Input: part model. Units: mm. Frame: model coordinates. A direction names the side the tool comes from. Coordinates: 2 decimals unless noted, no trailing zeros. Loops run counter-clockwise (first coordinate to the right, second up) from the corner with the lowest first, then second, coordinate; pieces in that order, holes last. Notation, with made-up numbers: (1, 16.5) - (26, 16.5) arc R19 ccw to (26, 26.5) - close; hole circle Ø4 at (83.25, -29.5). An arc over 180 degrees is marked (long way). Use one line per item in the form item = value.
from build123d import *

# Parameters (mm, degrees)
F0_W     = 660.4
F0_H     = 254
F1_DEPTH = 152.4
F2_W     = 654.05
F2_H     = 247.65
F3_DEPTH = 152.401
F4_W     = 685.8
F4_H     = 279.4
F4_W_2   = 660.4
F4_H_2   = 254
F5_DEPTH = 3.175
F6_R     = 9.525
F7_DEPTH = 3.175


with BuildPart() as f1:
    # F0 (on Top) → F1 (new body)
    with BuildSketch(Plane.XY):
        Rectangle(F0_W, F0_H)
    extrude(amount=F1_DEPTH)

    # F2 (on face) → F3 (cut, through all)
    with BuildSketch(Plane.XY.offset(152.4)):
        Rectangle(F2_W, F2_H)
    extrude(amount=-F3_DEPTH, mode=Mode.SUBTRACT)

    # F4 (on face) → F5 (join)
    with BuildSketch(Plane.XY.offset(152.4)):
        Rectangle(F4_W, F4_H)
        Rectangle(F4_W_2, F4_H_2, mode=Mode.SUBTRACT)
    extrude(amount=-F5_DEPTH)

    # F6 (on face) → F7 (cut, through all)
    with BuildSketch(Plane.XZ.offset(127)):
        with Locations((0, 25.4)):
            Circle(F6_R)
    extrude(amount=-F7_DEPTH, mode=Mode.SUBTRACT)


solid = f1.part
Q1. Set-up query: faces 1 (the flat face through (-5, 127, 74)), 2 (the flat face through (330.2, -2, 74)), 3 (the cylindrical face through (-2.06, -125.43, 16.1)), 4 (the flat face through (-327.025, -2, 77)). Return all of +Z, -Z, +X, -X, +Y, -Y with unobstructed straight access to the full face (end or side cutting, diameter ignored); none if empty.
Check values:
face_1 = -Z, +X, -X, +Y
face_2 = -Z, +X, +Y, -Y
face_3 = -Y
face_4 = +Z, -Z
Q2. Cut plane C-C, the plane x = 0. Return loops of the section in (y, z) (3 decimals).
Check values:
outline = (-139.7, 149.225) - (-127, 149.225) - (-127, 34.925) - (-123.825, 34.925) - (-123.825, 152.4) - (-139.7, 152.4) - close; (-127, 0) - (-123.825, 0) - (-123.825, 15.875) - (-127, 15.875) - close; (123.825, 0) - (127, 0) - (127, 149.225) - (139.7, 149.225) - (139.7, 152.4) - (123.825, 152.4) - close
Q3. Cut plane A-A, the plane y = 95. Return loops of the section in (x, z) (3 decimals).
Check values:
outline = (-342.9, 149.225) - (-330.2, 149.225) - (-330.2, 0) - (-327.025, 0) - (-327.025, 152.4) - (-342.9, 152.4) - close; (327.025, 0) - (330.2, 0) - (330.2, 149.225) - (342.9, 149.225) - (342.9, 152.4) - (327.025, 152.4) - close
Q4. Ray query, line 1 along Y through (x, z) = (76, 49.5) (3 decimals); line 2 along X through (y, z) = (-20, 90.5) (3 decimals); line 3 along Z through (x, y) = (0, -124.75) (3 decimals). Return the intervals inside material, ascending. Write a range as [from, to].
Check values:
line_1 = [-127, -123.825], [123.825, 127]
line_2 = [-330.2, -327.025], [327.025, 330.2]
line_3 = [0, 15.875], [34.925, 152.4]
Q5. Cut plane B-B, the plane x = 71.5. Return loops of the section in (y, z) (3 decimals), then the cut area to 3 significant figures.
Check values:
outline = (-139.7, 149.225) - (-127, 149.225) - (-127, 0) - (-123.825, 0) - (-123.825, 152.4) - (-139.7, 152.4) - close; (123.825, 0) - (127, 0) - (127, 149.225) - (139.7, 149.225) - (139.7, 152.4) - (123.825, 152.4) - close
area = 1,050 mm²
Q6. First-contact query: P1, Ø12, axis at x = -112, z = 86.5, coming from the -Y side; P2, Ø10, axis at y = 82, z = 104, coming from the +X side; P3, Ø17, axis at x = 0, z = 25.4, coming from the +Y side. Flat tips, straight axial feed; report the tip coordinate or a pass-through.
Check values:
P1 = -127
P2 = 330.2
P3 = 127
Q7. Pull-direction query (X, two-part tool) for faces 5 (the flat face through (-5, -127, 74)), 6 (the flat face through (-330.2, -2, 74)), 7 (the flat face through (327.025, -2, 77)); classes: pulls with the +X half, pulls with the -X half, needs draft (parallel to the pull), parting line crosses it, or undercut.
Check values:
face_5 = needs draft
face_6 = pulls with the -X half
face_7 = undercut
Q8. Cut plane D-D, the plane z = 113.5. Return loops of the section in (x, y) (3 decimals).
Check values:
outline = (-330.2, -127) - (330.2, -127) - (330.2, 127) - (-330.2, 127) - close; hole (-327.025, -123.825) - (327.025, -123.825) - (327.025, 123.825) - (-327.025, 123.825) - close
